from build123d import *

# Parameters (mm, degrees)
BOSS_EXTRUDE1_DEPTH = 14
FILLET2_R           = 45
SKETCH2_R           = 18.51
CUT_EXTRUDE1_DEPTH  = 15
SKETCH3_R           = 13.985
CUT_EXTRUDE2_DEPTH  = 7
BOSS_EXTRUDE2_DEPTH = 14
CUT_EXTRUDE3_DEPTH  = 101.407669397
CUT_EXTRUDE4_DEPTH  = 101.407669397
SKETCH9_R           = 20.51
SKETCH9_R_2         = 18.51
SKETCH9_R_3         = 15.985
SKETCH9_R_4         = 13.985
BOSS_EXTRUDE3_DEPTH = 4
FILLET5_R           = 2
SKETCH10_R          = 3.5
CUT_EXTRUDE5_DEPTH  = 42
SKETCH11_R          = 3.5
CUT_EXTRUDE6_DEPTH  = 42
CUT_EXTRUDE7_DEPTH  = 42


with BuildPart() as part:
    # Sketch1 → Boss-Extrude1 (new body)
    with BuildSketch(Plane(origin=(0, 0, 0), x_dir=(1, 0, 0), z_dir=(0, 1, 0))):
        with BuildLine():
            Line((-103.75, -33.919328315), (-11.25, 19.485571585))
            ThreePointArc((-11.25, 19.485571585), (0, 22.5), (11.25, 19.485571585))
            Line((11.25, 19.485571585), (103.75, -33.919328315))
            ThreePointArc((103.75, -33.919328315), (111.985571585, -64.6548999), (81.25, -72.890471485))
            Line((81.25, -72.890471485), (0, -25.980762114))
            Line((0, -25.980762114), (-81.25, -72.890471485))
            ThreePointArc((-81.25, -72.890471485), (-111.985571585, -64.6548999), (-103.75, -33.919328315))
        make_face()
    extrude(amount=BOSS_EXTRUDE1_DEPTH)

    # Fillet2
    fillet2_edges = [part.edges().sort_by_distance(p)[0] for p in [
        (0, 7, 25.980762114),
    ]]
    fillet(fillet2_edges, radius=FILLET2_R)

    # Sketch2 → Cut-Extrude1 (cut, through all)
    with BuildSketch(Plane(origin=(0, 14, 0), x_dir=(1, 0, 0), z_dir=(0, 1, 0))):
        with Locations((-92.5, -53.4048999)):
            Circle(SKETCH2_R)
        with Locations((92.5, -53.4048999)):
            Circle(SKETCH2_R)
    extrude(amount=-CUT_EXTRUDE1_DEPTH, mode=Mode.SUBTRACT)

    # Sketch3 → Cut-Extrude2 (cut)
    with BuildSketch(Plane(origin=(0, 14, 0), x_dir=(1, 0, 0), z_dir=(0, 1, 0))):
        Circle(SKETCH3_R)
    extrude(amount=-CUT_EXTRUDE2_DEPTH, mode=Mode.SUBTRACT)

    # Sketch4 → Boss-Extrude2 (add)
    with BuildSketch(Plane(origin=(0, 14, 0), x_dir=(1, 0, 0), z_dir=(0, 1, 0))):
        with BuildLine():
            Line((-114.523687548, -48.799773759), (-131.844195624, -58.799773759))
            Line((-131.844195624, -58.799773759), (-116.844195624, -84.780535872))
            Line((-116.844195624, -84.780535872), (-99.523687548, -74.780535872))
            ThreePointArc((-99.523687548, -74.780535872), (-111.985571585, -64.6548999), (-114.523687548, -48.799773759))
        make_face()
        with BuildLine():
            Line((114.523687548, -48.799773759), (131.844195624, -58.799773759))
            Line((131.844195624, -58.799773759), (116.844195624, -84.780535872))
            Line((116.844195624, -84.780535872), (99.523687548, -74.780535872))
            ThreePointArc((99.523687548, -74.780535872), (111.985571585, -64.6548999), (114.523687548, -48.799773759))
        make_face()
    extrude(amount=-BOSS_EXTRUDE2_DEPTH)

    # Sketch5 → Cut-Extrude3 (cut, through all)
    with BuildSketch(Plane(origin=(7.5, 0, 12.990381057), x_dir=(0.866025404, 0, -0.5), z_dir=(0.5, 0, 0.866025404))):
        with BuildLine():
            Line((-143.580309631, 0), (-143.580309631, 14))
            Line((-143.580309631, 14), (-134.580309631, 14))
            ThreePointArc((-134.580309631, 14), (-141.580309631, 7), (-134.580309631, 0))
            Line((-134.580309631, 0), (-143.580309631, 0))
        make_face()
    extrude(amount=-CUT_EXTRUDE3_DEPTH, mode=Mode.SUBTRACT)

    # Sketch6 → Cut-Extrude4 (cut, through all)
    with BuildSketch(Plane(origin=(-7.5, 0, 12.990381057), x_dir=(0.866025404, 0, 0.5), z_dir=(-0.5, 0, 0.866025404))):
        with BuildLine():
            Line((134.580309631, 14), (143.580309631, 14))
            Line((143.580309631, 14), (143.580309631, 0))
            Line((143.580309631, 0), (134.580309631, 0))
            ThreePointArc((134.580309631, 0), (141.580309631, 7), (134.580309631, 14))
        make_face()
    extrude(amount=-CUT_EXTRUDE4_DEPTH, mode=Mode.SUBTRACT)

    # Sketch9 → Boss-Extrude3 (add)
    with BuildSketch(Plane(origin=(0, 14, 0), x_dir=(1, 0, 0), z_dir=(0, 1, 0))):
        with Locations((-92.5, -53.4048999)):
            Circle(SKETCH9_R)
        with Locations((-92.5, -53.4048999)):
            Circle(SKETCH9_R_2, mode=Mode.SUBTRACT)
        Circle(SKETCH9_R_3)
        Circle(SKETCH9_R_4, mode=Mode.SUBTRACT)
        with Locations((92.5, -53.4048999)):
            Circle(SKETCH9_R)
        with Locations((92.5, -53.4048999)):
            Circle(SKETCH9_R_2, mode=Mode.SUBTRACT)
    extrude(amount=BOSS_EXTRUDE3_DEPTH)

    # Fillet5
    fillet5_edges = [part.edges().sort_by_distance(p)[0] for p in [
        (-113.01, 14, 53.4048999),
        (-15.985, 14, 0),
        (71.99, 14, 53.4048999),
    ]]
    fillet(fillet5_edges, radius=FILLET5_R)

    # Sketch10 → Cut-Extrude5 (cut)
    with BuildSketch(Plane(origin=(7.5, 0, 12.990381057), x_dir=(0.866025404, 0, -0.5), z_dir=(0.5, 0, 0.866025404))):
        with Locations((-134.580309631, 7)):
            Circle(SKETCH10_R)
    extrude(amount=-CUT_EXTRUDE5_DEPTH, mode=Mode.SUBTRACT)

    # Sketch11 → Cut-Extrude6 (cut)
    with BuildSketch(Plane(origin=(-7.5, 0, 12.990381057), x_dir=(0.866025404, 0, 0.5), z_dir=(-0.5, 0, 0.866025404))):
        with Locations((134.580309631, 7)):
            Circle(SKETCH11_R)
    extrude(amount=-CUT_EXTRUDE6_DEPTH, mode=Mode.SUBTRACT)

    # Sketch12 → Cut-Extrude7 (cut)
    with BuildSketch(Plane(origin=(0, 18, 0), x_dir=(1, 0, 0), z_dir=(0, 1, 0))):
        Polygon((-92.363302775, -53.614217526), (-129.001019076, -74.767012895), (-129.274413527, -74.348377643), (-92.636697225, -53.195582274), align=None)
        Polygon((129.274413527, -74.348377643), (129.001019076, -74.767012895), (92.363302775, -53.614217526), (92.636697225, -53.195582274), align=None)
    extrude(amount=-CUT_EXTRUDE7_DEPTH, mode=Mode.SUBTRACT)


solid = part.part
Input: part model. Units: mm. Frame: model coordinates. A direction names the side the tool comes from. Coordinates: 2 decimals unless noted, no trailing zeros. Loops run counter-clockwise (first coordinate to the right, second up) from the corner with the lowest first, then second, coordinate; pieces in that order, holes last.
(1) Section B-B on x = 0. Return the cut outline in (y, z) (3 decimals), then the cut area to 3 significant figures.
(2) Section A-A on z = 0. Return the cut outline in (x, y) (3 decimals), then the cut area to 3 significant figures.
(3) Set-up query: faces 1 (the face through (112.41, 7.13, 65.19)), 2 (the face through (75.204, 16.986, 42.382)), 3 (the face through (-51.46, 6.9, 55.69)), 4 (the face through (118.75, 6.85, 77.48)), 5 (the face through (-110, 14, 72)). Return all of +Z, -Z, +X, -X, +Y, -Y with unobstructed straight access to the full face (end or side cutting, diameter ignored); none if empty.
(4) Pull-direction query (Y, two-part tool) for faces 6 (the face through (-111.287, 3.895, 73.175)), 7 (the face through (-96, 18, 35)), 8 (the face through (13.34, 12.42, -4.2)), 9 (the face through (117.905, 4.87, 59.388)); classes: released by +Y, released by -Y, zero draft, split by the parting line, or undercut.
(5) Material intervals for probe 1 along X at (y, z) = (4.75, 67.5); probe 2 along X at (y, z) = (13, 37); probe 3 along X at (y, z) = (10, 58), sorted ascending.
(6) First-contact query: pin 1 Ø4 at (x, y) = (-72.5, 6.5) entering from +Z; pin 2 Ø6 at (x, y) = (-29, 13) entering from -Z; pin 3 Ø1.5 at (y, z) = (6.5, 35) entering from -X; pin 4 Ø22 at (x, z) = (92.5, 53.4) entering from +Y. Flat tips, straight axial feed; report the tip coordinate or a pass-through.
(7) Section C-C on x = -32. Return the cut outline in (y, z), then the cut area to 3 significant figures.
Data:
1. outline: (0, -22.5) - (14, -22.5) - (14, -17.985) arc R2 cw to (16, -15.985) - (18, -15.985) - (18, -13.985) - (7, -13.985) - (7, 13.985) - (18, 13.985) - (18, 15.985) - (16, 15.985) arc R2 cw to (14, 17.985) - (14, 32.942) - (0, 32.942) - close
1. area: 598 mm2
2. outline: (-45, 0) - (45, 0) - (45, 14) - (17.985, 14) arc R2 cw to (15.985, 16) - (15.985, 18) - (13.985, 18) - (13.985, 7) - (-13.985, 7) - (-13.985, 18) - (-15.985, 18) - (-15.985, 16) arc R2 cw to (-17.985, 14) - (-45, 14) - close
2. area: 1,080 mm2
3. face 1: +Y, -Y
3. face 2: +Y
3. face 3: +Z, +Y, -Y
3. face 4: +Z, +X
3. face 5: +Z, -X, +Y
4. face 6: undercut
4. face 7: released by +Y
4. face 8: zero draft
4. face 9: undercut
5. probe 1: x = -124.08 to -119.52, -113.33 to -104.5, -80.5 to -71.91, 71.91 to 80.5, 104.5 to 113.33, 119.52 to 124.08
5. probe 2: x = -107.9 to -101.07, -83.93 to -18.67, 18.67 to 83.93, 101.07 to 107.9
5. probe 3: x = -129.22 to -124, -119.83 to -110.43, -74.57 to -55.46, 55.46 to 74.57, 110.43 to 119.83, 124 to 129.22
6. pin 1: stops at z = 68.99
6. pin 2: stops at z = -10.97
6. pin 3: stops at x = -106.45
6. pin 4: passes through
7. outline: (0, -7.51) - (14, -7.51) - (14, 44.46) - (0, 44.46) - close
7. area: 727 mm2
